Here's how the part is built. I have some questions about the finished solid (model axes, mm). A direction names the side the tool comes from. Give positions to 0.01 mm unless a question says otherwise; leave off trailing zeros. Loops run counter-clockwise (first coordinate to the right, second up) from the corner with the lowest first, then second, coordinate; pieces in that order, holes last.
Q1. Suppose I cut it at B-B (z = 0.8). Count the separate pieces of the cut face and the enclosed holes in it, and give its area (3 significant figures).
Q2. I need wall thicknesses on probe 1 along X at (y, z) = (179, 0.25); probe 2 along Y at (x, z) = (-6.5, 0.7); probe 3 along Y at (x, z) = (-3, 1.5). Which ranges of each line are inside material? Lowest first, please.
Q3. Thinking about a two-plate mould opening in X: for faces 3 (the face through (37.675, -50.7, 0.986)), 4 (the face through (-2.059, 290.726, 0.986)), 5 (the face through (18, 107, 2)), 6 (the face through (-37.325, -49.3, 0.986)), which applies, pulls with the +X half, pulls with the -X half, needs draft (parallel to the pull), parting line crosses it, or undercut?
Q4. I'm going to push flat-ended pins straight in: P1, Ø0.6, axis at y = 228, z = 1, coming from the -X side; P2, Ø1, axis at y = -34.5, z = 0.5, coming from the -X side; P3, Ø2.5, axis at x = 0, y = -57.5, coming from the +Z side; P4, Ø0.6, axis at y = 128.5, z = 1, coming from the +X side. Where does each tip first touch, or does it pass through?
Q5. For faces 1 (the face through (0.33, 161.148, 0.986)), 2 (the face through (0.55, 324.994, 0.986)), which set-ups out of +Z, -Z, +X, -X, +Y, -Y let a thin tool reach every point of the face, with its end or its side?
Q6. Suppose I cut it at A-A (y = 74.5). List the corners of the cut face in (x, z) for me.
```python
from build123d import *

# Parameters (mm, degrees)
SKETCH_1_R      = 2
SKETCH_1_R_2    = 2.08
SKETCH_1_R_3    = 5
SKETCH_1_R_4    = 9.5
EXTRUDE_1_DEPTH = 2


with BuildPart() as part:
    # 草图1 → 凸台-拉伸1 (new body)
    with BuildSketch(Plane.XY):
        with BuildLine():
            Line((37.188144312, -109.964533236), (48.296291314, -112.940952255))
            ThreePointArc((48.296291314, -112.940952255), (49.572243069, -106.526309611), (50, -100))
            Line((50, -100), (25, 0))
            Line((25, 0), (25, 300))
            ThreePointArc((25, 300), (0, 325), (-25, 300))
            Line((-25, 300), (-25, 0))
            Line((-25, 0), (-50, -100))
            ThreePointArc((-50, -100), (-49.572243069, -106.526309611), (-48.296291314, -112.940952255))
            Line((-48.296291314, -112.940952255), (-37.188144312, -109.964533236))
            ThreePointArc((-37.188144312, -109.964533236), (0, -61.5), (37.188144312, -109.964533236))
        make_face()
        with Locations((0, -15)):
            Circle(SKETCH_1_R, mode=Mode.SUBTRACT)
        with Locations((-12.990381057, -7.5)):
            Circle(SKETCH_1_R, mode=Mode.SUBTRACT)
        with Locations((-12.990381057, 7.5)):
            Circle(SKETCH_1_R, mode=Mode.SUBTRACT)
        with Locations((0, 15)):
            Circle(SKETCH_1_R, mode=Mode.SUBTRACT)
        with Locations((12.990381057, 7.5)):
            Circle(SKETCH_1_R, mode=Mode.SUBTRACT)
        with Locations((12.990381057, -7.5)):
            Circle(SKETCH_1_R, mode=Mode.SUBTRACT)
        with Locations((-13.53, 0)):
            Circle(SKETCH_1_R_2, mode=Mode.SUBTRACT)
        with Locations((6.765, 11.717323713)):
            Circle(SKETCH_1_R_2, mode=Mode.SUBTRACT)
        with Locations((6.765, -11.717323713)):
            Circle(SKETCH_1_R_2, mode=Mode.SUBTRACT)
        Circle(SKETCH_1_R_3, mode=Mode.SUBTRACT)
        with Locations((-42.5, -100)):
            Circle(SKETCH_1_R, mode=Mode.SUBTRACT)
        with Locations((-30.0520382, -69.9479618)):
            Circle(SKETCH_1_R, mode=Mode.SUBTRACT)
        with Locations((0, -57.5)):
            Circle(SKETCH_1_R, mode=Mode.SUBTRACT)
        with Locations((30.0520382, -69.9479618)):
            Circle(SKETCH_1_R, mode=Mode.SUBTRACT)
        with Locations((42.5, -100)):
            Circle(SKETCH_1_R, mode=Mode.SUBTRACT)
        with Locations((0, 300)):
            Circle(SKETCH_1_R_4, mode=Mode.SUBTRACT)
        with BuildLine():
            Line((-15, 37.231839261), (-15, 138.190211212))
            ThreePointArc((-15, 138.190211212), (0, 153.190211212), (15, 138.190211212))
            Line((15, 138.190211212), (15, 37.231839261))
            ThreePointArc((15, 37.231839261), (0, 22.231839261), (-15, 37.231839261))
        make_face(mode=Mode.SUBTRACT)
        with BuildLine():
            Line((-7.285756476, -21.115181502), (7.285756476, -21.115181502))
            ThreePointArc((7.285756476, -21.115181502), (22.853925458, -36.683350484), (7.285756476, -52.251519465))
            Line((7.285756476, -52.251519465), (-7.285756476, -52.251519465))
            ThreePointArc((-7.285756476, -52.251519465), (-22.853925458, -36.683350484), (-7.285756476, -21.115181502))
        make_face(mode=Mode.SUBTRACT)
        with BuildLine():
            Line((-15, 176.144279665), (-15, 268.287785105))
            ThreePointArc((-15, 268.287785105), (0, 283.287785105), (15, 268.287785105))
            Line((15, 268.287785105), (15, 176.144279665))
            ThreePointArc((15, 176.144279665), (0, 161.144279665), (-15, 176.144279665))
        make_face(mode=Mode.SUBTRACT)
    extrude(amount=EXTRUDE_1_DEPTH)


solid = part.part
```
Solutions:
1. separate pieces: 1
1. enclosed holes: 19
1. area: 12,500 mm2
2. probe 1: x = -25 to -15, 15 to 25
2. probe 2: y = -62.05 to -52.25, -21.12 to 23.71, 151.71 to 162.63, 281.81 to 293.07, 306.93 to 324.14
2. probe 3: y = -61.62 to -52.25, -21.12 to -4, 4 to 22.53, 152.89 to 161.45, 282.98 to 290.99, 309.01 to 324.82
3. face 3: pulls with the +X half
3. face 4: undercut
3. face 5: needs draft
3. face 6: pulls with the -X half
4. P1: stops at x = -25
4. P2: stops at x = -33.75
4. P3: passes through
4. P4: stops at x = 25
5. face 1: +Z, -Z
5. face 2: +Z, -Z, +Y
6. outline: (-25, 0) - (-15, 0) - (-15, 2) - (-25, 2) - close; (15, 0) - (25, 0) - (25, 2) - (15, 2) - close
